Geometry: see drawing. Coordinates: mm, zero at the bounding-box minimum. Coordinates: 2 decimals unless noted, no trailing zeros. Loops run counter-clockwise (first coordinate to the right, second up) from the corner with the lowest first, then second, coordinate; pieces in that order, holes last. Notation, with made-up numbers: M 28,-39.5 L 48,-39.5 A13 cw 48,-31.5 Z; hole C 53.5,-7.5 d3. An arc over 180 degrees is marked long. One line per question, with ' | ' between items. Start each with the question number.
1. Section query A-A, the plane x = 70. Output: boundary loops of the cut face in (y, z).
2. Ray query, probe 1 along X at (y, z) = (4.5, 2.3); probe 2 along X at (y, z) = (6, 2.65); probe 3 along Y at (x, z) = (70, 3). Return the intervals inside material, ascending.
3. Section query B-B, the plane z = 0.8. Output: boundary loops of the cut face in (x, y), and give its area (3 significant figures).
4. Section query C-C, the plane y = 4.25. Output: boundary loops of the cut face in (x, z).
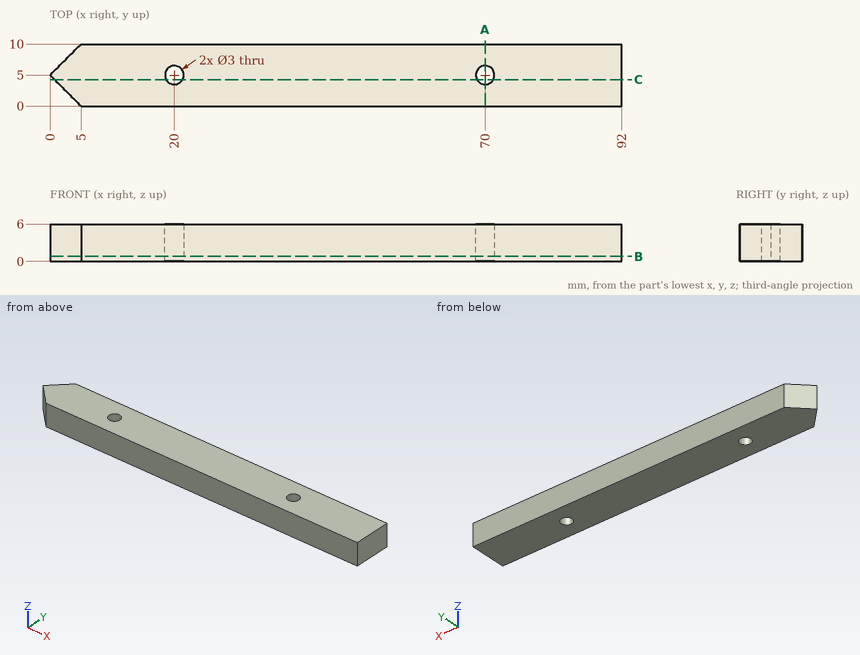
Taken from the geometry:
1) outline: M 0,0 L 3.5,0 L 3.5,6 L 0,6 Z; M 6.5,0 L 10,0 L 10,6 L 6.5,6 Z
2) probe 1: 0.5 to 18.59, 21.41 to 68.59, 71.41 to 92 | probe 2: 1 to 18.88, 21.12 to 68.88, 71.12 to 92 | probe 3: 0 to 3.5, 6.5 to 10
3) outline: M 0,5 L 5,0 L 92,0 L 92,10 L 5,10 Z; hole C 20,5 d3; hole C 70,5 d3 | area: 881 mm^2
4) outline: M 0.75,0 L 18.7,0 L 18.7,6 L 0.75,6 Z; M 21.3,0 L 68.7,0 L 68.7,6 L 21.3,6 Z; M 71.3,0 L 92,0 L 92,6 L 71.3,6 Z
